Answer from the drawing. Dimensions are ordinates in mm from the lowest x, y and z of the part. A direction names the side the tool comes from. Give positions to 0.01 mm unless a question says otherwise; leave off trailing zeros. Write each loop counter-clockwise with the first axis right and the second up, starting at its lowest first coordinate (ties: lowest second). Pieces come first, ordered by that corner, then holes. Notation, with made-up numbers: M 33,-32 L 86,-32 A28 ccw 86,4 Z; hole C 81,64.25 d10. An arc over 180 degrees is marked long. Put each result on its own line as item: value.
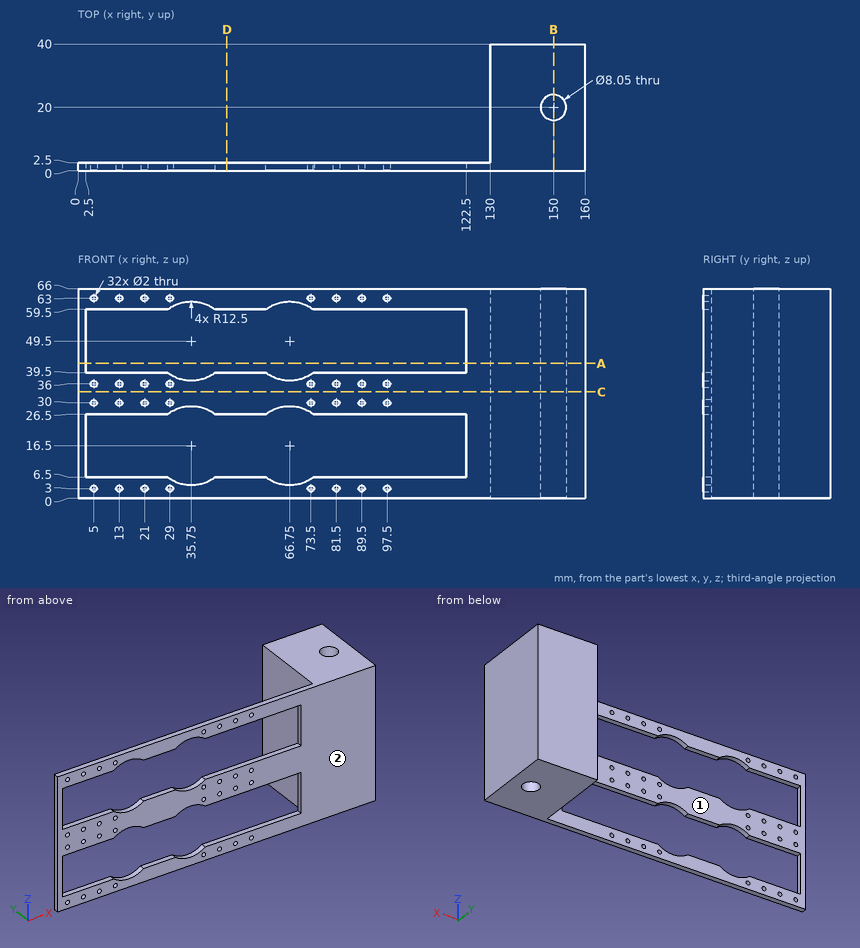
(1) Section D-D on x = 47 is taken. Determine the outline of the cut face in (y, z), and give its area (3 significant figures).
Result:
outline: M 0,0 L 2.5,0 L 2.5,6.5 L 0,6.5 Z; M 0,26.5 L 2.5,26.5 L 2.5,39.5 L 0,39.5 Z; M 0,59.5 L 2.5,59.5 L 2.5,66 L 0,66 Z
area: 65.0 mm²
(2) Section B-B on x = 150 is taken. Determine the outline of the cut face in (y, z) (3 decimals).
Result:
outline: M 0,0 L 15.975,0 L 15.975,66 L 0,66 Z; M 24.025,0 L 40,0 L 40,66 L 24.025,66 Z
(3) Given pin 1 Ø1.5 at (y, z) = (21.5, 29.5) entering from -X; pin 2 Ø1.2 at (x, z) = (21, 3) entering from +Y; pin 3 Ø0.8 at (x, y) = (54.5, 1) entering from -Z; pin 4 Ø3 at (x, z) = (89.5, 63) entering from +Y, each flat-ended and moving along its own axis, determine where each tip first touches the part or whether it passes through.
Result:
pin 1: stops at x = 130
pin 2: passes through
pin 3: stops at z = 0
pin 4: stops at y = 2.5
(4) Which of the six approach directions +Z, -Z, +X, -X, +Y, -Y give full straight-line access (tool end or side, diameter ignored) to the marked faces 1 and 2?
Result:
face 1: +Z, -Z, -X, +Y
face 2: +Z, -Z, +X, -X, -Y
(5) Straight lines are drawn through the part: line 1 along X through (y, z) = (28.5, 62); line 2 along X through (y, z) = (21, 53); line 3 along Y through (x, z) = (121.5, 36). For each, find the intervals that lie inside material, in ascending order. Write a range as from..to.
Result:
line 1: x = 130..160
line 2: x = 130..146.1, 153.9..160
line 3: y = 0..2.5
(6) Section A-A on z = 42.5 is taken. Determine the outline of the cut face in (x, y) (3 decimals), and give its area (3 significant figures).
Result:
outline: M 0,0 L 2.5,0 L 2.5,2.5 L 0,2.5 Z; M 122.5,0 L 160,0 L 160,40 L 130,40 L 130,2.5 L 122.5,2.5 Z; hole C 150,20 d8.05
area: 1,170 mm²
(7) Section C-C on z = 33.5 is taken. Determine the outline of the cut face in (x, y) (3 decimals), and give its area (3 significant figures).
Result:
outline: M 0,0 L 160,0 L 160,40 L 130,40 L 130,2.5 L 0,2.5 Z; hole C 150,20 d8.05
area: 1,470 mm²
